from build123d import *

# Parameters (mm, degrees)
SKETCH1_R               = 62.5
BOSS_EXTRUDE1_DEPTH     = 175
CUT_EXTRUDE1_START      = -1.5
SKETCH2_R               = 59.5
CUT_EXTRUDE1_DEPTH      = 172
SKETCH3_R               = 25
BOSS_EXTRUDE2_DEPTH     = 20
SKETCH4_R               = 22
CUT_EXTRUDE2_DEPTH      = 30
FILLET1_R               = 0.75
SKETCH5_R               = 17.5
CUT_EXTRUDE3_DEPTH      = 63.5000001
CUT_EXTRUDE3_DEPTH_BACK = 70


with BuildPart() as part:
    # Sketch1 → Boss-Extrude1 (new body)
    with BuildSketch(Plane(origin=(0, 0, 0), x_dir=(1, 0, 0), z_dir=(0, 1, 0))):
        Circle(SKETCH1_R)
    extrude(amount=BOSS_EXTRUDE1_DEPTH)

    # Sketch2 → Cut-Extrude1 (cut)
    with BuildSketch(Plane(origin=(0, 175, 0), x_dir=(1, 0, 0), z_dir=(0, 1, 0)).offset(CUT_EXTRUDE1_START)):
        Circle(SKETCH2_R)
    extrude(amount=-CUT_EXTRUDE1_DEPTH, mode=Mode.SUBTRACT)

    # Sketch3 → Boss-Extrude2 (add)
    with BuildSketch(Plane(origin=(0, 175, 0), x_dir=(1, 0, 0), z_dir=(0, 1, 0))):
        Circle(SKETCH3_R)
    extrude(amount=BOSS_EXTRUDE2_DEPTH)

    # Sketch4 → Cut-Extrude2 (cut)
    with BuildSketch(Plane(origin=(0, 195, 0), x_dir=(1, 0, 0), z_dir=(0, 1, 0))):
        Circle(SKETCH4_R)
    extrude(amount=-CUT_EXTRUDE2_DEPTH, mode=Mode.SUBTRACT)

    # Fillet1
    fillet1_edges = [part.edges().sort_by_distance(p)[0] for p in [
        (-25, 175, 0),
        (-25, 195, 0),
        (-22, 195, 0),
        (-62.5, 0, 0),
        (-62.5, 175, 0),
    ]]
    fillet(fillet1_edges, radius=FILLET1_R)

    # Sketch5 → Cut-Extrude3 (cut, two sides)
    with BuildSketch(Plane.XY) as cut_extrude3_sk:
        with Locations((0, 44.895186866)):
            Circle(SKETCH5_R)
    extrude(amount=CUT_EXTRUDE3_DEPTH, mode=Mode.SUBTRACT)
    extrude(cut_extrude3_sk.sketch, amount=-CUT_EXTRUDE3_DEPTH_BACK, mode=Mode.SUBTRACT)


solid = part.part
Part model, mm, in its own coordinate system. A direction names the side the tool comes from. Coordinates: 2 decimals unless noted, no trailing zeros. Order: outer loops, then holes, each group sorted by start corner. A loop starts at its lowest first (then second) coordinate and runs counter-clockwise, first axis right, second up.
(1) Slice it at A-A, the plane x = 0. State how many separate pieces and enclosed holes the cut face has, and give its area (3 significant figures).
Check sheet entries:
separate pieces: 3
enclosed holes: 0
area: 1,250 mm2
(2) Pull direction Z, two halves, no side cores. Call faces 4 (the face through (-1, 0, -1)), 5 (the face through (57.734, 86.286, 23.938)), 6 (the face through (27.456, 88.704, 52.787)): pulls with the +Z half, pulls with the -Z half, needs draft (parallel to the pull), parting line crosses it, or undercut.
Check sheet entries:
face 4: needs draft
face 5: parting line crosses it
face 6: undercut
(3) Slice it at B-B, the plane y = 99.5. Write the cut outline in (x, z).
Check sheet entries:
outline: circle Ø125 at (0, 0); hole circle Ø119 at (0, 0)
(4) Probe L1, parallel to Y at x = -28, z = -27; L2, parallel to Z at x = 0, y = 182. List the from-to ranges inside material, lowest first.
Check sheet entries:
L1: y = 0 to 1.5, 173.5 to 175
L2: z = -25 to -22, 22 to 25
(5) Pin check, flat tips, straight feed: pin 1 Ø3 at (y, z) = (60, -6) entering from -X; pin 2 Ø1 at (x, y) = (-27, 149) entering from -Z; pin 3 Ø1 at (x, z) = (-26.5, 34) entering from +Y. Stop position of each tip, or through.
Check sheet entries:
pin 1: stops at x = -62.34
pin 2: stops at z = -56.6
pin 3: stops at y = 175
(6) Tool access for faces 1 (the face through (26, 173.5, -1)), 2 (the face through (23.846, 184.87, -7.509)), 3 (the face through (7, 195, -22)): list every direction of +Z, -Z, +X, -X, +Y, -Y with a clear straight run to the whole face (end or side of a thin tool).
Check sheet entries:
face 1: none
face 2: +Y
face 3: +Z, -Z, +X, -X, +Y
